For this review, take the finished solid that the model builds, in its own axes (mm). A direction names the side the tool comes from. Round coordinates to 2 decimals unless told otherwise and drop trailing zeros. Write each loop counter-clockwise with the first axis right and the second up, starting at its lowest first coordinate (ties: lowest second). Pieces come first, ordered by that corner, then holes. Notation, with made-up numbers: M 39.5,85 L 57.5,85 A11 ccw 57.5,99 Z; hole C 78,4.5 d11. An arc over 180 degrees is marked long. Use one line per item in the form item = value. Start each with the question number.
Item 1: For faces 5 (the flat face through (0, 10.835, -2)), 6 (the flat face through (0, 12.422, -1)), 7 (the cylindrical face through (-17.46, -13.94, -2.35)), 8 (the cylindrical face through (17.46, 13.94, -2.35)), list the 3-axis set-ups (+Z, -Z, +X, -X, +Y, -Y) from which the entire face can be reached by the end or side of a thin tool; tool diameter is ignored.
Item 2: Add section A-A (z = -1). Count the separate pieces of the cut face and the enclosed holes in it, and give its area (3 significant figures).
Item 3: Add section D-D (x = 0). State the section outline as (y, z) points (1 decimal).
Item 4: For line 1 (Y direction, x = -4, z = -1.25) (1 decimal); line 2 (Y direction, x = -1, z = 1.75); line 3 (Y direction, x = 18.5, z = 1), list the stretches that pass through material, from the lowest coordinate up. Write a range as [from, to].
Item 5: Add section B-B (x = 18.5). State the section outline as (y, z) points, and give its area (3 significant figures).
Item 6: Draft analysis for pull direction X (two halves, no side actions). For faces 1 (the cylindrical face through (23.9, -19.45, 1.01)), 2 (the cylindrical face through (-23.9, 19.45, 1.01)), 3 (the cylindrical face through (15.875, -13.975, -1.429)), 4 (the flat face through (0, 0, 0)), state which applies: released by +X, released by -X, zero draft, split by the parting line, or undercut.
Item 7: For P1, Ø4, axis at x = 0.5, z = -3.5, coming from the -Y side (3 decimals); P2, Ø12, axis at x = -8.5, y = -9, coming from the -Z side; P3, Ø1, axis at x = 6.5, z = -3.5, coming from the +Y side (3 decimals); P4, Ø2, axis at x = -16, z = -1.5, coming from the +Y side, all flat-tipped, find the tip position at first contact; note any pin that passes through.
Autodesk Inventor part; units mm, degrees
ref_plane "YZ Plane" through (0, 0, 0) normal (1, 0, 0) x (0, 1, 0)
ref_plane "XZ Plane" through (0, 0, 0) normal (0, 1, 0) x (-1, 0, 0)
ref_plane "XY Plane" through (0, 0, 0) normal (0, 0, 1) x (1, 0, 0)
sketch "Sketch1" plane through (0, 0, 0) normal (0, 0, 1) x (1, 0, 0)
  line L0 (-24.85, -20.36) -> (24.85, -20.36)
  line L1 (24.85, -20.36) -> (24.85, 20.36)
  line L2 (24.85, 20.36) -> (-24.85, 20.36)
  line L3 (-24.85, 20.36) -> (-24.85, -20.36)
  line L4 (-24.85, -20.36) -> (24.85, 20.36) construction
  line L5 (24.85, -20.36) -> (-24.85, 20.36) construction
  point P0 (0, 0)
  dimension "d0" = 49.7
  dimension "d1" = 40.72
extrude "Extrusion1" add sketch "Sketch1" along normal blind 2
sketch "Sketch3" plane through (0, 0, 0) normal (0, 0, -1) x (-1, 0, 0)
  line L0 (24.85, 20.36) -> (24.85, -20.36)
  line L1 (14.2875, -14.01) -> (-14.2875, -14.01) construction
  line L2 (14.2875, -10.835) -> (-14.2875, -10.835)
  line L3 (-14.2875, -17.185) -> (14.2875, -17.185)
  arc A0 (14.2875, -17.185) -> (14.2875, -10.835) centre (14.2875, -14.01) ccw
  arc A1 (-14.2875, -10.835) -> (-14.2875, -17.185) centre (-14.2875, -14.01) ccw
  line L4 (0, -28.504) -> (0, 28.504)
  line L5 (34.79, 0) -> (-34.79, 0)
  line L6 (14.2875, 14.01) -> (-14.2875, 14.01) construction
  line L7 (14.2875, 17.185) -> (-14.2875, 17.185)
  line L8 (-14.2875, 10.835) -> (14.2875, 10.835)
  arc A2 (14.2875, 10.835) -> (14.2875, 17.185) centre (14.2875, 14.01) ccw
  arc A3 (-14.2875, 17.185) -> (-14.2875, 10.835) centre (-14.2875, 14.01) ccw
  point P0 (0, 0)
  point P1 (0, -14.01)
  point P2 (0, 14.01)
  dimension "d28" = 3.175
  dimension "d29" = 28.02
  dimension "d30" = 28.575
sketch "Sketch5" plane through (0, 0, 0) normal (0, 0, -1) x (-1, 0, 0)
  line L0 (0, -28.504) -> (0, 28.504)
  line L1 (34.79, 0) -> (-34.79, 0)
  point P0 (0, 0)
  point P1 (-18.5, 7.9375)
  point P2 (18.5, 7.9375)
  dimension "d17" = 37
  dimension "d26" = 7.9375
hole "Hole1" at (18.5, 7.9375, 0) at (-18.5, 7.9375, 0) direction (0, 0, 1) diameter 3 depth 2
fillet "Fillet1" radius 3.175 4 edges at (24.85, -20.36, 1) (24.85, 20.36, 1) (-24.85, 20.36, 1) (-24.85, -20.36, 1)
extrude "Extrusion4" add sketch "Sketch3" along normal blind 4.7625
sketch "Sketch6" plane through (0, 0, -4.7625) normal (0, 0, -1) x (-1, 0, 0)
  line L0 (14.2875, -10.835) -> (-14.2875, -10.835)
  arc A0 (-14.2875, -10.835) -> (-14.2875, -17.185) centre (-14.2875, -14.01) ccw
  line L1 (-14.2875, -17.185) -> (14.2875, -17.185)
  arc A1 (14.2875, -17.185) -> (14.2875, -10.835) centre (14.2875, -14.01) ccw
  line L2 (14.2875, 17.185) -> (-14.2875, 17.185)
  arc A2 (-14.2875, 17.185) -> (-14.2875, 10.835) centre (-14.2875, 14.01) ccw
  line L3 (-14.2875, 10.835) -> (14.2875, 10.835)
  arc A3 (14.2875, 10.835) -> (14.2875, 17.185) centre (14.2875, 14.01) ccw
  line L4 (14.2875, -14.01) -> (-14.2875, -14.01) construction
  line L5 (14.2875, -12.4225) -> (-14.2875, -12.4225)
  line L6 (-14.2875, -15.5975) -> (14.2875, -15.5975)
  arc A4 (14.2875, -15.5975) -> (14.2875, -12.4225) centre (14.2875, -14.01) ccw
  arc A5 (-14.2875, -12.4225) -> (-14.2875, -15.5975) centre (-14.2875, -14.01) ccw
  line L7 (14.2875, 14.01) -> (-14.2875, 14.01) construction
  line L8 (14.2875, 15.5975) -> (-14.2875, 15.5975)
  line L9 (-14.2875, 12.4225) -> (14.2875, 12.4225)
  arc A6 (14.2875, 12.4225) -> (14.2875, 15.5975) centre (14.2875, 14.01) ccw
  arc A7 (-14.2875, 15.5975) -> (-14.2875, 12.4225) centre (-14.2875, 14.01) ccw
  point P0 (0, 0)
  point P1 (0, -14.01)
  point P2 (0, 14.01)
  dimension "d33" = 1.5875
extrude "Extrusion5" cut sketch "Sketch6" along normal through all both and the other way through all contours A4 L6 A5 L5 | A6 L9 A7 L8
properties part number "RC_CAR_ARDUINO_PLATE"
Calculated:
q1.face_5 = -Z, +X, -X
q1.face_6 = +Z, -Z
q1.face_7 = -Z, -X
q1.face_8 = -Z, +X
q2.separate_pieces = 2
q2.enclosed_holes = 2
q2.area = 229 mm^2
q3.outline = M -20.4,0 L -17.2,0 L -17.2,-4.8 L -15.6,-4.8 L -15.6,2 L -20.4,2 Z; M -12.4,-4.8 L -10.8,-4.8 L -10.8,0 L 10.8,0 L 10.8,-4.8 L 12.4,-4.8 L 12.4,2 L -12.4,2 Z; M 15.6,-4.8 L 17.2,-4.8 L 17.2,0 L 20.4,0 L 20.4,2 L 15.6,2 Z
q4.line_1 = [-17.2, -15.6], [-12.4, -10.8], [10.8, 12.4], [15.6, 17.2]
q4.line_2 = [-20.36, -15.6], [-12.42, 12.42], [15.6, 20.36]
q4.line_3 = [-20.36, 6.44], [9.44, 20.36]
q5.outline = M -20.36,0 L 6.44,0 L 6.44,2 L -20.36,2 Z; M 9.44,0 L 20.36,0 L 20.36,2 L 9.44,2 Z
q5.area = 75.4 mm^2
q6.face_1 = released by +X
q6.face_2 = released by -X
q6.face_3 = undercut
q6.face_4 = zero draft
q7.P1 = -17.185
q7.P2 = -4.76
q7.P3 = 17.185
q7.P4 = 17.1
